from build123d import *

# Parameters (mm, degrees)
ESQUISSE1_R                  = 40
BOSS_EXTRU_1_DEPTH           = 20
ENL_V_START                  = 20
ESQUISSE2_R                  = 31.25
ENL_V_MAT_EXTRU_1_DEPTH      = 18
CONG_3_R                     = 1
ESQUISSE4_W                  = 80
ESQUISSE4_H                  = 80
BOSS_EXTRU_2_DEPTH           = 3
ENL_V_MAT_EXTRU_2_DEPTH      = 61
ENL_V_MAT_EXTRU_2_DEPTH_BACK = 61
ESQUISSE5_R                  = 17.5
D_GAGEMENT_M41_D             = 4.3
SYM_TRIE2_COPY_1_D           = 4.3


with BuildPart() as part:
    # Esquisse1 → Boss.-Extru.1 (new body)
    with BuildSketch(Plane.XY):
        Circle(ESQUISSE1_R)
    extrude(amount=BOSS_EXTRU_1_DEPTH)

    # Esquisse2 → Enlèv. mat.-Extru.1 (cut)
    with BuildSketch(Plane.XY.offset(ENL_V_START)):
        Circle(ESQUISSE2_R)
    extrude(amount=-ENL_V_MAT_EXTRU_1_DEPTH, mode=Mode.SUBTRACT)

    # Congé3
    cong_3_edges = [part.edges().sort_by_distance(p)[0] for p in [
        (-31.25, 0, 2),
    ]]
    fillet(cong_3_edges, radius=CONG_3_R)

    # Esquisse4 → Boss.-Extru.2 (add)
    with BuildSketch(Plane.XY):
        Rectangle(ESQUISSE4_W, ESQUISSE4_H)
    extrude(amount=-BOSS_EXTRU_2_DEPTH)

    # Esquisse5 → Enlèv. mat.-Extru.2 (cut, two sides: drawn at the far end of the back side and taken through both)
    with BuildSketch(Plane.XY.offset(-ENL_V_MAT_EXTRU_2_DEPTH_BACK)):
        Circle(ESQUISSE5_R)
    extrude(amount=ENL_V_MAT_EXTRU_2_DEPTH + ENL_V_MAT_EXTRU_2_DEPTH_BACK, mode=Mode.SUBTRACT)

    # Dégagement M41 (through all)
    with Locations(Plane(origin=(-36, 36, 0), x_dir=(1, 0, 0), z_dir=(0, 0, 1))):
        with Locations((0, 0)):
            d_gagement_m41 = Hole(D_GAGEMENT_M41_D / 2)

    # Symétrie1: Dégagement M41 across plane
    add(d_gagement_m41.mirror(Plane(origin=(0, 0, 0), x_dir=(0, 0, 1), z_dir=(1, 0, 0))), mode=Mode.SUBTRACT)

    # Symétrie2: Dégagement M41 across plane
    add(d_gagement_m41.mirror(Plane.ZX), mode=Mode.SUBTRACT)

    # Symétrie2 copy 1 (through all)
    with Locations(Plane(origin=(36, -36, 0), x_dir=(-1, 0, 0), z_dir=(0, 0, 1))):
        with Locations((0, 0)):
            Hole(SYM_TRIE2_COPY_1_D / 2)


solid = part.part
Design review of the part built by this model. Coordinates are the model's own, in mm. A direction names the side the tool comes from. Coordinates: 2 decimals unless noted, no trailing zeros. Order: outer loops, then holes, each group sorted by start corner. A loop starts at its lowest first (then second) coordinate and runs counter-clockwise, first axis right, second up. Notation, with made-up numbers: M 51.5,13 L 106.5,13 A21 ccw 106.5,26 Z; hole C -20,13 d9. An arc over 180 degrees is marked long. Use a Markdown table: item, result.
(1) Wall thickness on probe 1 along Y at (x, z) = (36, -2.35); probe 2 along Y at (x, z) = (0, 12.75); probe 3 along Z at (x, y) = (24, 34.5): over which ranges is each line inside the solid? List them lowest first.
Worked answers:
| item | result |
|---|---|
| probe 1 | y = -40 to -38.15, -33.85 to 33.85, 38.15 to 40 |
| probe 2 | y = -40 to -31.25, 31.25 to 40 |
| probe 3 | z = -3 to 0 |
(2) For P1, Ø5.5, axis at x = 36, y = 36, coming from the +Z side; P2, Ø6, axis at x = -26.5, z = 12.5, coming from the -Y side; P3, Ø8, axis at x = 14.5, y = 7.5, coming from the +Z side, all flat-tipped, find the tip position at first contact; note any pin that passes through.
Worked answers:
| item | result |
|---|---|
| P1 | stops at z = 0 |
| P2 | stops at y = -32.37 |
| P3 | stops at z = 2 |
(3) Draft analysis for pull direction X (two halves, no side actions). For faces 1 (the flat face through (30, 30, 0)), 2 (the flat face through (40, -1, -1)), 3 (the flat face through (-40, -1, -1)), 4 (the cylindrical face through (-13.887, -10.648, -0.535)), state which applies: released by +X, released by -X, zero draft, split by the parting line, or undercut.
Worked answers:
| item | result |
|---|---|
| face 1 | zero draft |
| face 2 | released by +X |
| face 3 | released by -X |
| face 4 | undercut |
(4) Add section A-A (x = 36). Give the boundary of the cut face in (y, z).
Worked answers:
| item | result |
|---|---|
| outline | M -40,-3 L -38.15,-3 L -38.15,0 L -40,0 Z; M -33.85,-3 L 33.85,-3 L 33.85,0 L 17.44,0 L 17.44,20 L -17.44,20 L -17.44,0 L -33.85,0 Z; M 38.15,-3 L 40,-3 L 40,0 L 38.15,0 Z |
(5) Add section C-C (z = 6.5). Give the boundary of the cut face in (x, y).
Worked answers:
| item | result |
|---|---|
| outline | C 0,0 d80; hole C 0,0 d62.5 |
(6) For faces 5 (the flat face through (-32, -30, 0)), 6 (the cylindrical face through (-31.22, 1.37, 11.62)), 7 (the flat face through (-30, 32, 0)), list the 3-axis set-ups (+Z, -Z, +X, -X, +Y, -Y) from which the entire face can be reached by the end or side of a thin tool; tool diameter is ignored.
Worked answers:
| item | result |
|---|---|
| face 5 | +Z, -X, -Y |
| face 6 | +Z |
| face 7 | +Z, -X, +Y |
